Autodesk Inventor part; units mm, degrees
ref_plane "YZ Plane" through (0, 0, 0) normal (1, 0, 0) x (0, 1, 0)
ref_plane "XZ Plane" through (0, 0, 0) normal (0, 1, 0) x (-1, 0, 0)
ref_plane "XY Plane" through (0, 0, 0) normal (0, 0, 1) x (1, 0, 0)
sketch "Sketch1" plane through (0, 0, 0) normal (0, 1, 0) x (-1, 0, 0)
  line L0 (13.2677, 19.6408) -> (-12.1323, 19.6408)
  line L1 (-12.1323, 19.6408) -> (-12.1323, -18.4592)
  line L2 (-12.1323, -18.4592) -> (13.2677, -18.4592)
  line L3 (13.2677, -18.4592) -> (13.2677, 19.6408)
  point P0 (0, 0)
  dimension "d0" = 25.4
  dimension "d1" = 38.1
extrude "Extrusion1" add sketch "Sketch1" along normal blind 3.175
hole "Hole1" at (-9.6799, 3.175, 14.8783) direction (0, -1, 0) diameter 4.4958 depth 3.175
hole "Hole2" at (8.5446, 3.175, 14.8783) direction (0, -1, 0) diameter 4.4958 depth 3.175
hole "Hole3" at (-9.6799, 3.175, -13.6967) direction (0, -1, 0) diameter 4.4958 depth 3.175
hole "Hole4" at (8.5446, 3.175, -13.6967) direction (0, -1, 0) diameter 4.4958 depth 3.175
sketch "Sketch2" plane through (0, 3.175, 0) normal (0, 1, 0) x (1, 0, 0)
  circle A0 centre (0, 0) radius 3.175
  dimension "d58" = 6.35
extrude "Extrusion2" add sketch "Sketch2" along normal blind 304.8
sketch "Sketch3" plane through (0, 0, 0) normal (1, 0, 0) x (0, 1, 0)
  point P0 (0, 0)
sketch "Sketch4" plane through (0, 307.975, 0) normal (0, 1, 0) x (1, 0, 0)
  circle A0 centre (0, 0) radius 3.175
extrude "Extrusion3" add sketch "Sketch4" along normal blind 63.5
sketch "Sketch5" plane through (0, 0, 0) normal (1, 0, 0) x (0, 1, 0)
  point P0 (0, 0)
properties part number "rotatable rod table"
Here's how the part is built. I have some questions about the finished solid (model axes, mm). A direction names the side the tool comes from. Coordinates: 2 decimals unless noted, no trailing zeros. Loops run counter-clockwise (first coordinate to the right, second up) from the corner with the lowest first, then second, coordinate; pieces in that order, holes last.
1. For faces 1 (the flat face through (0, 371.475, 0)), 2 (the cylindrical face through (-0.69, 184.75, -3.1)), which set-ups out of +Z, -Z, +X, -X, +Y, -Y let a thin tool reach every point of the face, with its end or its side?
2. Imagine slicing it at A-A, the plane z = 0. Please give me the cut outline in (x, y) (3 decimals), and give its area (3 significant figures).
3. Imagine slicing it at B-B, the plane x = 0. Please give me the cut outline in (y, z) (3 decimals).
4. Imagine slicing it at C-C, the plane y = 174.5. Please give me the cut outline in (x, z) (3 decimals).
5. I need wall thicknesses on L1, parallel to Y at x = -12, z = 5 (3 decimals); L2, parallel to Z at x = 0.5, y = 338; L3, parallel to Z at x = 1.5, y = 318. Which ranges of each line are inside material? Lowest first, please.
6. For P1, Ø1, axis at x = 1, y = 46.5, coming from the +Z side; P2, Ø1.5, axis at x = -10, z = -1, coming from the +Y side (3 decimals); P3, Ø12, axis at x = -6, y = 42, coming from the +Z side (3 decimals), each with a flat end and sliding along its axis, tell me the tip position at first contact or that it passes through.
Taken from the geometry:
1. face 1: +Z, -Z, +X, -X, +Y
1. face 2: +Y
2. outline: (-13.268, 0) - (12.132, 0) - (12.132, 3.175) - (3.175, 3.175) - (3.175, 371.475) - (-3.175, 371.475) - (-3.175, 3.175) - (-13.268, 3.175) - close
2. area: 2,420 mm2
3. outline: (0, -18.459) - (3.175, -18.459) - (3.175, -3.175) - (371.475, -3.175) - (371.475, 3.175) - (3.175, 3.175) - (3.175, 19.641) - (0, 19.641) - close
4. outline: circle Ø6.35 at (0, 0)
5. L1: y = 0 to 3.175
5. L2: z = -3.14 to 3.14
5. L3: z = -2.8 to 2.8
6. P1: stops at z = 3.14
6. P2: stops at y = 3.175
6. P3: stops at z = 3.175
